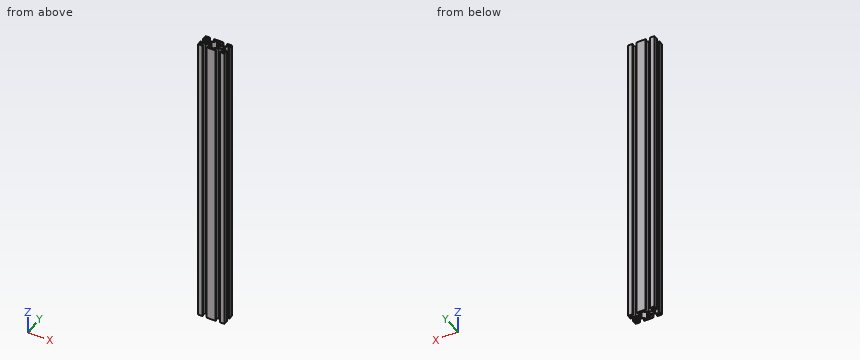
from build123d import *

# Parameters (mm, degrees)
F0_R     = 2.5
F1_DEPTH = 450


with BuildPart() as f1:
    # F0 (on Top) → F1 (new body)
    with BuildSketch(Plane.XY):
        Polygon((6.5, 7.616114), (1.4, 2.389949), (1.4, 6.8), (0, 6.8), (0, 0), (6.8, 0), (6.8, 1.4), (2.389949, 1.4), (7.489949, 6.5), (12.510051, 6.5), (17.610051, 1.4), (13.2, 1.4), (13.2, 0), (20, 0), (26.8, 0), (26.8, 1.4), (22.389949, 1.4), (27.489949, 6.5), (32.510051, 6.5), (37.610051, 1.4), (33.2, 1.4), (33.2, 0), (40, 0), (40, 6.8), (38.6, 6.8), (38.6, 2.389949), (33.5, 7.489949), (33.5, 12.510051), (38.6, 17.610051), (38.6, 13.2), (40, 13.2), (40, 20), (33.2, 20), (33.2, 18.6), (37.610051, 18.6), (32.510051, 13.5), (27.489949, 13.5), (22.389949, 18.6), (26.8, 18.6), (26.8, 20), (20, 20), (13.2, 20), (13.2, 18.6), (17.610051, 18.6), (12.510051, 13.5), (7.489949, 13.5), (2.389949, 18.6), (6.8, 18.6), (6.8, 20), (0, 20), (0, 13.2), (1.4, 13.2), (1.4, 17.610051), (6.5, 12.510051), align=None)
        with Locations((10, 10)):
            Circle(F0_R, mode=Mode.SUBTRACT)
        Polygon((13.5, 7.489949), (13.5, 12.510051), (18.6, 17.610051), (21.4, 17.610051), (26.5, 12.510051), (26.5, 7.616114), (21.4, 2.389949), (18.6, 2.389949), align=None, mode=Mode.SUBTRACT)
        with Locations((30, 10)):
            Circle(F0_R, mode=Mode.SUBTRACT)
    extrude(amount=F1_DEPTH)


solid = f1.part
Geometry check sheet. Reference: the model listing, model coordinates, mm. Round coordinates to 2 decimals unless told otherwise and drop trailing zeros. Answer in a Markdown table with one row per item.
(1) Go/stop test with flat-tipped pins: P1, Ø4, axis at y = 9, z = 314, coming from the +X side; P2, Ø1.5, axis at y = 9, z = 153.5, coming from the +X side; P3, Ø2, axis at x = 15.5, y = 9.5, coming from the +Z side; P4, Ø1.5, axis at x = 10.5, z = 198.5, coming from the +Y side. Record where each tip stops, or that it passes through.
Responses:
| item | result |
|---|---|
| P1 | stops at x = 33.99 |
| P2 | stops at x = 33.5 |
| P3 | passes through |
| P4 | stops at y = 13.5 |
(2) Scan lines: probe 1 along X at (y, z) = (1, 149); probe 2 along Y at (x, z) = (30, 170); probe 3 along Y at (x, z) = (37, 136). Record each from-to range of solid material in increasing order. Write a range as from..to.
Responses:
| item | result |
|---|---|
| probe 1 | x = 0..6.8, 13.2..26.8, 33.2..40 |
| probe 2 | y = 6.5..7.5, 12.5..13.5 |
| probe 3 | y = 0..1.4, 2.01..3.99, 16.01..17.99, 18.6..20 |
(3) Sectioned sample at A-A, the plane z = 349.5. State how many separate pieces and enclosed holes the cut face has, and give its area (3 significant figures).
Responses:
| item | result |
|---|---|
| separate pieces | 1 |
| enclosed holes | 3 |
| area | 252 mm² |
